Geometry check sheet. Reference: the model listing, model coordinates, mm. Face numbers are marked on the shaded views. A direction names the side the tool comes from. Give positions to 0.01 mm unless a question says otherwise; leave off trailing zeros. Loops run counter-clockwise (first coordinate to the right, second up) from the corner with the lowest first, then second, coordinate; pieces in that order, holes last.
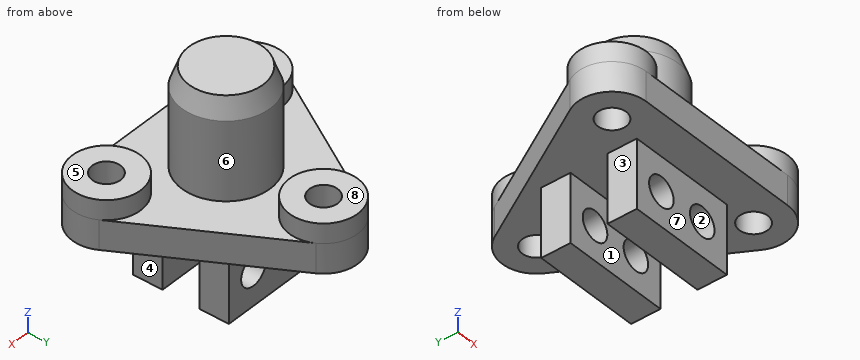
```python
from build123d import *

# Parameters (mm, degrees)
SKETCH_R      = 1.45
PAD_DEPTH     = 3
SKETCH001_W   = 11
SKETCH001_H   = 3
PAD001_DEPTH  = 7
SKETCH002_R   = 1.5
POCKET_DEPTH  = 9.8
SKETCH003_R   = 3.5
SKETCH003_R_2 = 1.45
PAD002_DEPTH  = 2
SKETCH004_R   = 4.525
PAD003_DEPTH  = 10
CHAMFER_ANGLE = 20
CHAMFER_SIZE  = 2


with BuildPart() as part:
    # Sketch → Pad (new body)
    with BuildSketch(Plane.XY):
        with BuildLine():
            ThreePointArc((3.031089, 11.75), (0, 13.5), (-3.031089, 11.75))
            Line((-11.691343, -3.25), (-3.031089, 11.75))
            ThreePointArc((-11.691343, -3.25), (-11.691343, -6.75), (-8.660254, -8.5))
            Line((8.660254, -8.5), (-8.660254, -8.5))
            ThreePointArc((8.660254, -8.5), (11.691343, -6.75), (11.691343, -3.25))
            Line((3.031089, 11.75), (11.691343, -3.25))
        make_face()
        with Locations((0, 10)):
            Circle(SKETCH_R, mode=Mode.SUBTRACT)
        with Locations((8.660254, -5)):
            Circle(SKETCH_R, mode=Mode.SUBTRACT)
        with Locations((-8.660254, -5)):
            Circle(SKETCH_R, mode=Mode.SUBTRACT)
    extrude(amount=PAD_DEPTH)

    # Sketch001 (on Face10 of Pad) → Pad001 (join)
    with BuildSketch(Plane(origin=(0, 0, 0), x_dir=(1, 0, 0), z_dir=(0, 0, -1))):
        with Locations((0, 3.4)):
            Rectangle(SKETCH001_W, SKETCH001_H)
        with Locations((0, -3.4)):
            Rectangle(SKETCH001_W, SKETCH001_H)
    extrude(amount=PAD001_DEPTH)

    # Sketch002 (on Face18 of Pad001) → Pocket (cut)
    with BuildSketch(Plane(origin=(0, 4.9, 0), x_dir=(-1, 0, 0), z_dir=(0, 1, 0))):
        with Locations((-2.5, -3.5)):
            Circle(SKETCH002_R)
        with Locations((2.5, -3.5)):
            Circle(SKETCH002_R)
    extrude(amount=-POCKET_DEPTH, mode=Mode.SUBTRACT)

    # Sketch003 (on Face5 of Pocket) → Pad002 (join)
    with BuildSketch(Plane.XY.offset(3)):
        with Locations((0, 10)):
            Circle(SKETCH003_R)
        with Locations((0, 10)):
            Circle(SKETCH003_R_2, mode=Mode.SUBTRACT)
        with Locations((8.660254, -5)):
            Circle(SKETCH003_R)
        with Locations((8.660254, -5)):
            Circle(SKETCH003_R_2, mode=Mode.SUBTRACT)
        with Locations((-8.660254, -5)):
            Circle(SKETCH003_R)
        with Locations((-8.660254, -5)):
            Circle(SKETCH003_R_2, mode=Mode.SUBTRACT)
    extrude(amount=PAD002_DEPTH)

    # Sketch004 (on Face4 of Pad002) → Pad003 (join)
    with BuildSketch(Plane.XY.offset(3)):
        Circle(SKETCH004_R)
    extrude(amount=PAD003_DEPTH)

    # Chamfer
    chamfer_edges = [part.edges().sort_by_distance(p)[0] for p in [
        (-4.525, 0, 13),
    ]]
    chamfer_side = part.faces().sort_by_distance((-4.525, 0, 8))[0]
    chamfer(chamfer_edges, length=CHAMFER_SIZE, angle=CHAMFER_ANGLE, reference=chamfer_side)


solid = part.part
```
1) Sectioned sample at A-A on x = 0. Enter the section's corners in (y, z) (3 decimals), plus the area to 3 significant figures.
2) Mould release check, pull along X, two halves, no side actions. Record for the marked faces 1, 2, 3 and 4: +X half, -X half, draft (parallel to the pull), parting line (faces both ways), or undercut.
3) Sectioned sample at D-D on y = 10. Enter the section's corners in (x, z), plus the area to 3 significant figures.
4) Sectioned sample at C-C on y = -5.75. Enter the section's corners in (x, z), plus the area to 3 significant figures.
5) Tool access check on the marked faces 5, 6, 7 and 8. Record the directions out of +Z, -Z, +X, -X, +Y, -Y that give a thin tool (end or side, any length) a straight path to the whole face; none if there is none.
6) Depth check by flat-ended pin: P1, Ø2.5, axis at y = 3, z = -3.5, coming from the +X side; P2, Ø2, axis at x = -10, y = -4.5, coming from the +Z side; P3, Ø2.5, axis at y = -3.5, z = -3, coming from the -X side; P4, Ø7.5, axis at x = 0.5, z = -3.5, coming from the +Y side. Enter the tip coordinate at first touch or a pass-through.
7) Sectioned sample at B-B on z = -3.5. Enter the section's corners in (x, y), plus the area to 3 significant figures.
8) Scan lines: line 1 along Z through (x, y) = (-2.5, 3.9); line 2 along Y through (x, z) = (-0.5, 4.75); line 3 along X through (y, z) = (4.25, -4.5). Record each from-to range of solid material in increasing order.
Determined:
1. outline: (-8.5, 0) - (-4.9, 0) - (-4.9, -7) - (-1.9, -7) - (-1.9, 0) - (1.9, 0) - (1.9, -7) - (4.9, -7) - (4.9, 0) - (8.55, 0) - (8.55, 5) - (6.5, 5) - (6.5, 3) - (4.525, 3) - (4.525, 11) - (3.797, 13) - (-3.797, 13) - (-4.525, 11) - (-4.525, 3) - (-8.5, 3) - close; (11.45, 0) - (13.5, 0) - (13.5, 5) - (11.45, 5) - close
1. area: 197 mm2
2. face 1: draft
2. face 2: undercut
2. face 3: -X half
2. face 4: +X half
3. outline: (-4.04, 0) - (-1.45, 0) - (-1.45, 5) - (-3.5, 5) - (-3.5, 3) - (-4.04, 3) - close; (1.45, 0) - (4.04, 0) - (4.04, 3) - (3.5, 3) - (3.5, 5) - (1.45, 5) - close
3. area: 23.7 mm2
4. outline: (-12.08, 0) - (-9.9, 0) - (-9.9, 5) - (-12.08, 5) - close; (-7.42, 0) - (7.42, 0) - (7.42, 5) - (5.24, 5) - (5.24, 3) - (-5.24, 3) - (-5.24, 5) - (-7.42, 5) - close; (9.9, 0) - (12.08, 0) - (12.08, 5) - (9.9, 5) - close
4. area: 75.0 mm2
5. face 5: +Z, +X, +Y, -Y
5. face 6: +Z
5. face 7: -Z, +X, -X, -Y
5. face 8: +Z, +X, -X, +Y
6. P1: stops at x = 5.5
6. P2: stops at z = 5
6. P3: stops at x = -5.5
6. P4: stops at y = 13.5
7. outline: (-5.5, -4.9) - (-4, -4.9) - (-4, -1.9) - (-5.5, -1.9) - close; (-5.5, 1.9) - (-4, 1.9) - (-4, 4.9) - (-5.5, 4.9) - close; (-1, -4.9) - (1, -4.9) - (1, -1.9) - (-1, -1.9) - close; (-1, 1.9) - (1, 1.9) - (1, 4.9) - (-1, 4.9) - close; (4, -4.9) - (5.5, -4.9) - (5.5, -1.9) - (4, -1.9) - close; (4, 1.9) - (5.5, 1.9) - (5.5, 4.9) - (4, 4.9) - close
7. area: 30.0 mm2
8. line 1: z = -7 to -5, -2 to 3
8. line 2: y = -4.5 to 4.5, 6.54 to 8.64, 11.36 to 13.46
8. line 3: x = -5.5 to -3.62, -1.38 to 1.38, 3.62 to 5.5
